Geometry: final body of the model. Coordinates: model frame, mm. Face numbers are marked on the shaded views. A direction names the side the tool comes from. Give positions to 0.01 mm unless a question says otherwise; leave off trailing zeros. Write each loop counter-clockwise with the first axis right and the second up, starting at its lowest first coordinate (ties: lowest second). Pieces come first, ordered by that corner, then holes. Notation, with made-up numbers: M -1,88.25 L 16,88.25 A20 ccw 16,102.25 Z; hole C -32,77 d5. An arc over 180 degrees is marked long. Use a Markdown table: item, result. Add a question column.
(1) Reachability of the marked faces 1, 2 and 3 from +Z, -Z, +X, -X, +Y, -Y: full face, straight path, thin tool, end or side. Return the list, or none.
(2) Draft query along Y for the marked faces 4, 5 and 6. Return one class per face: released by +Y, released by -Y, zero draft, split by the parting line, or undercut.
(3) Pin query (flat end, axial travel): pin 1 Ø1 at (x, y) = (0.5, 4.5) entering from +Z; pin 2 Ø3 at (y, z) = (6.5, 2) entering from -X (3 decimals); pin 3 Ø2 at (x, y) = (0, 2.5) entering from -Z. Return the tip coordinate at first contact, or that it passes through.
(4) Cut plane D-D (y = 4.5). Output: boundary loops of the cut face in (x, z), plus the area to 3 significant figures.
(5) Cut plane A-A (x = 2.2). Output: boundary loops of the cut face in (y, z), plus the area to 3 significant figures.
(6) Material intervals for L1, parallel to Y at x = 1.65, z = 2.3; L2, parallel to X at y = 6.25, z = 1.2; L3, parallel to Z at x = 1.2, y = 0.25, sorted ascending.
(7) Cut plane B-B (y = 1). Output: boundary loops of the cut face in (x, z).
(8) Cut plane C-C (z = 2.1). Output: boundary loops of the cut face in (x, y), plus the area to 3 significant figures.
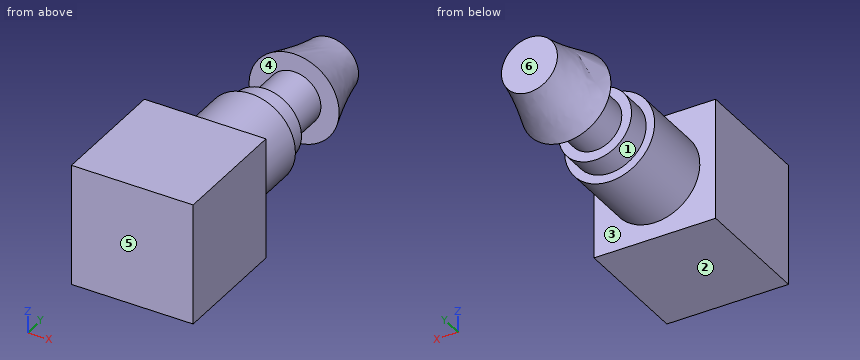
```python
from build123d import *

# Parameters (mm, degrees)
SKETCH1_R           = 1.85
BOSS_EXTRUDE1_DEPTH = 3.1
SKETCH2_R           = 1.5
BOSS_EXTRUDE2_DEPTH = 1
SKETCH3_R           = 1.1
BOSS_EXTRUDE3_DEPTH = 2
SKETCH6_W           = 5
SKETCH6_H           = 5
BOSS_EXTRUDE4_DEPTH = 5


with BuildPart() as part:
    # Sketch1 → Boss-Extrude1 (new body)
    with BuildSketch(Plane(origin=(0, 0, 0), x_dir=(1, 0, 0), z_dir=(0, 1, 0))):
        with Locations(Location((0, 0, 0), (0, 0, 90))):
            Circle(SKETCH1_R)
    extrude(amount=BOSS_EXTRUDE1_DEPTH)

    # Sketch2 → Boss-Extrude2 (add)
    with BuildSketch(Plane(origin=(0, 3.1, 0), x_dir=(1, 0, 0), z_dir=(0, 1, 0))):
        with Locations(Location((0, 0, 0), (0, 0, 270))):
            Circle(SKETCH2_R)
    extrude(amount=BOSS_EXTRUDE2_DEPTH)

    # Sketch3 → Boss-Extrude3 (add)
    with BuildSketch(Plane(origin=(0, 4.1, 0), x_dir=(1, 0, 0), z_dir=(0, 1, 0))):
        with Locations(Location((0, 0, 0), (0, 0, 270))):
            Circle(SKETCH3_R)
    extrude(amount=BOSS_EXTRUDE3_DEPTH)

    # Loft1: read off the stored shape, not the designer's step
    # Loft1: loft between two sections, ruled curve by curve
    loft1_from = [
        Edge.make_bspline([(0, 6.1, 1.85), (3.7, 6.1, 1.85), (3.7, 6.1, -1.85), (0, 6.1, -1.85), (-3.7, 6.1, -1.85), (-3.7, 6.1, 1.85), (0, 6.1, 1.85)], [0, 0, 0, 0, 0.5, 0.5, 0.5, 1, 1, 1, 1], 3, [1, 0.333333333, 0.333333333, 1, 0.333333333, 0.333333333, 1]),
    ]
    loft1_to = [
        Edge.make_bspline([(0.620465421, 8.6, 0.968257539), (2.556980499, 8.6, -0.272673303), (1.316049657, 8.6, -2.209188381), (-0.620465421, 8.6, -0.968257539), (-2.556980499, 8.6, 0.272673303), (-1.316049657, 8.6, 2.209188381), (0.620465421, 8.6, 0.968257539)], [0, 0, 0, 0, 0.5, 0.5, 0.5, 1, 1, 1, 1], 3, [1, 0.333333333, 0.333333333, 1, 0.333333333, 0.333333333, 1]),
    ]
    loft1 = Solid(Shell([*[Face.make_surface_from_curves(loft1_from[k], loft1_to[k]) for k in range(1)], Face(Wire(loft1_from)), Face(Wire(loft1_to))]))
    add(loft1)

    # Sketch6 → Boss-Extrude4 (add)
    with BuildSketch(Plane.XZ):
        Rectangle(SKETCH6_W, SKETCH6_H)
    extrude(amount=BOSS_EXTRUDE4_DEPTH)


solid = part.part
```
Answer list:
| question | item | result |
|---|---|---|
| 1 | face 1 | none |
| 1 | face 2 | -Z, +X, -X, +Y, -Y |
| 1 | face 3 | +Y |
| 2 | face 4 | undercut |
| 2 | face 5 | released by -Y |
| 2 | face 6 | released by +Y |
| 3 | pin 1 | z = 1.49 |
| 3 | pin 2 | x = -1.765 |
| 3 | pin 3 | z = -1.85 |
| 4 | outline | C 0,0 d2.2 |
| 4 | area | 3.80 mm² |
| 5 | outline | M -5,-2.5 L 0,-2.5 L 0,2.5 L -5,2.5 Z |
| 5 | area | 25.0 mm² |
| 6 | L1 | -5 to 0 |
| 6 | L2 | -1.34 to 1.34 |
| 6 | L3 | -1.41 to 1.41 |
| 7 | outline | C 0,0 d3.7 |
| 8 | outline | M -2.5,-5 L 2.5,-5 L 2.5,0 L -2.5,0 Z |
| 8 | area | 25.0 mm² |
